Build history of the part. All positions in model axes, mm. A direction names the side the tool comes from. Coordinates: 2 decimals unless noted, no trailing zeros. Loops run counter-clockwise (first coordinate to the right, second up) from the corner with the lowest first, then second, coordinate; pieces in that order, holes last.
(1) Slice it at A-A (y = -75). Give the cut face in (x, z).
(2) Tool access for faces 5 (the face through (-0.1, -29.5, -44.6)), 6 (the face through (-4.762, 1, 1)): list every direction of +Z, -Z, +X, -X, +Y, -Y with a clear straight run to the whole face (end or side of a thin tool).
(3) Slice it at B-B (z = -40). Give the cut face in (x, y), and give its area (3 significant figures).
(4) Flat gauge pins, fed straight in: P1, Ø5, axis at x = 1.5, y = -32, coming from the -Z side; P2, Ø1.5, axis at x = -3, z = -49.5, coming from the +Y side. Where does each tip first touch, or does it go through?
(5) Wall check: L1, parallel to Y at x = -1.5, z = -24.6; L2, parallel to Z at x = -2.5, y = 49; L3, parallel to Y at x = -3, z = -30. Give the ranges that are in metal, low to high.
(6) Two-plate mould, pull along X, no slides. Class faces 1 (the face through (0.06, -26.04, -33.36)), 2 (the face through (-0.325, -23.996, -39.53)), 3 (the face through (0, -19, 70)), 4 (the face through (4.762, 1, 1)): pulls with the +X half, pulls with the -X half, needs draft (parallel to the pull), parting line crosses it, or undercut.
(7) Slice it at C-C (y = 15). Give the cut face in (x, z), and give its area (3 significant figures).
from build123d import *

# Parameters (mm, degrees)
SKETCH1_W             = 9.525
SKETCH1_H             = 140
BOSS_EXTRUDE1_DEPTH   = 90
SKETCH3_R             = 14.29
SKETCH3_R_2           = 2.15
SKETCH3_R_3           = 14
CUT_EXTRUDE2_DEPTH    = 28.575
SKETCH5_W             = 25.4
SKETCH5_H             = 25.4
CUT_EXTRUDE4_DEPTH    = 10.525
M6_TAPPED_HOLE1_D     = 5
M6_TAPPED_HOLE1_DEPTH = 10
M6_TAPPED_HOLE1_TIP   = 1.502151548
M6_TAPPED_HOLE2_D     = 5
FILLET1_R             = 40


with BuildPart() as part:
    # Sketch1 → Boss-Extrude1 (new body, symmetric)
    with BuildSketch(Plane(origin=(0, 0, 0), x_dir=(1, 0, 0), z_dir=(0, 1, 0))):
        Rectangle(SKETCH1_W, SKETCH1_H)
    extrude(amount=BOSS_EXTRUDE1_DEPTH, both=True)

    # Sketch3 → Cut-Extrude2 (cut)
    with BuildSketch(Plane.ZY.offset(4.7625)):
        with Locations((-30, 50)):
            Circle(SKETCH3_R)
        with Locations((33.881108209, 27.347852166)):
            Circle(SKETCH3_R_2)
        with Locations((58.576812542, 27.347852166)):
            Circle(SKETCH3_R_2)
        with Locations((33.881108209, 2.652147834)):
            Circle(SKETCH3_R_2)
        with Locations((58.576812542, 2.652147834)):
            Circle(SKETCH3_R_2)
        with Locations((46.228960376, 15)):
            Circle(SKETCH3_R_3)
    extrude(amount=-CUT_EXTRUDE2_DEPTH, mode=Mode.SUBTRACT)

    # Sketch5 → Cut-Extrude4 (cut, through all)
    with BuildSketch(Plane.ZY.offset(4.7625)):
        with Locations((-57.3, -26.4746)):
            Rectangle(SKETCH5_W, SKETCH5_H)
    extrude(amount=-CUT_EXTRUDE4_DEPTH, mode=Mode.SUBTRACT)

    # M6 Tapped Hole1
    with Locations(Plane(origin=(0, 0, -44.6), x_dir=(-1, 0, 0), z_dir=(0, 0, -1))):
        with Locations((0, -26.4746)):
            Hole(M6_TAPPED_HOLE1_D / 2, depth=M6_TAPPED_HOLE1_DEPTH)
            with Locations((0, 0, -(M6_TAPPED_HOLE1_DEPTH + M6_TAPPED_HOLE1_TIP / 2))):  # 118° drill point
                Cone(0, M6_TAPPED_HOLE1_D / 2, M6_TAPPED_HOLE1_TIP, mode=Mode.SUBTRACT)

    # M6 Tapped Hole2 (through all)
    with Locations(Plane.ZY.offset(4.7625)):
        with Locations((-24.6, -28.7746), (55, -28.7746), (-24.6, -75), (55, -75)):
            Hole(M6_TAPPED_HOLE2_D / 2)

    # Fillet1
    fillet1_edges = [part.edges().sort_by_distance(p)[0] for p in [
        (0, 90, 70),
        (0, 90, -70),
    ]]
    fillet(fillet1_edges, radius=FILLET1_R)


solid = part.part
Response values:
1. outline: (-4.76, -70) - (4.76, -70) - (4.76, -27.1) - (-4.76, -27.1) - close; (-4.76, -22.1) - (4.76, -22.1) - (4.76, 52.5) - (-4.76, 52.5) - close; (-4.76, 57.5) - (4.76, 57.5) - (4.76, 70) - (-4.76, 70) - close
2. face 5: -Z, +X, -X
2. face 6: +Z, -Z, -X, +Y, -Y
3. outline: (-4.76, -90) - (4.76, -90) - (4.76, 39.79) - (-4.76, 39.79) - close; (-4.76, 60.21) - (4.76, 60.21) - (4.76, 88.73) - (-4.76, 88.73) - close; hole circle Ø5 at (0, -26.47)
3. area: 1,490 mm2
4. P1: stops at z = -44.6
4. P2: stops at y = 85.33
5. L1: y = -90 to -77.5, -72.5 to -31.27, -26.27 to 36.77, 63.23 to 90
5. L2: z = -70 to -44.25, -15.75 to 70
5. L3: y = -90 to 35.71, 64.29 to 90
6. face 1: undercut
6. face 2: undercut
6. face 3: needs draft
6. face 4: pulls with the +X half
7. outline: (-4.76, -70) - (4.76, -70) - (4.76, 32.23) - (-4.76, 32.23) - close; (-4.76, 60.23) - (4.76, 60.23) - (4.76, 70) - (-4.76, 70) - close
7. area: 1,070 mm2
